For this review, take the finished solid that the model builds, in its own axes (mm). Coordinates: 2 decimals unless noted, no trailing zeros. Loops run counter-clockwise (first coordinate to the right, second up) from the corner with the lowest first, then second, coordinate; pieces in that order, holes last. Notation, with made-up numbers: (-23.75, 26) - (-13.75, 26) arc R16 ccw to (-13.75, 53) - close; hole circle Ø5 at (12, -12). An arc over 180 degrees is marked (long way). One line per item, written item: value. Start each with the question number.
1. Insertion check: pin 1 (4 mm diameter, centred on y = 66.5, z = -1.5, fed in from -X); pin 2 (4 mm diameter, centred on x = -78, z = -1.5, fed in from +Y); pin 3 (1.5 mm diameter, centred on x = -76, z = -1.5, fed in from -Y). Each pin has a flat end and moves straight along its axis. Give the tip position at first contact, or say it passes through.
2. To check wall thickness, follow line 1 (Y direction, x = -69, z = -4); line 2 (Y direction, x = -26, z = -4); line 3 (Z direction, x = 11, y = -23). State the ranges of each line that lie inside material, in increasing order. Write a range as from..to.
3. Take a section at B-B, the plane y = -48.5. State the section outline as (x, z) points.
4. Take a section at C-C, the plane y = 38.5. State the section outline as (x, z) points, and give its area (3 significant figures).
5. Take a section at A-A, the plane x = 58. State the section outline as (y, z) points.
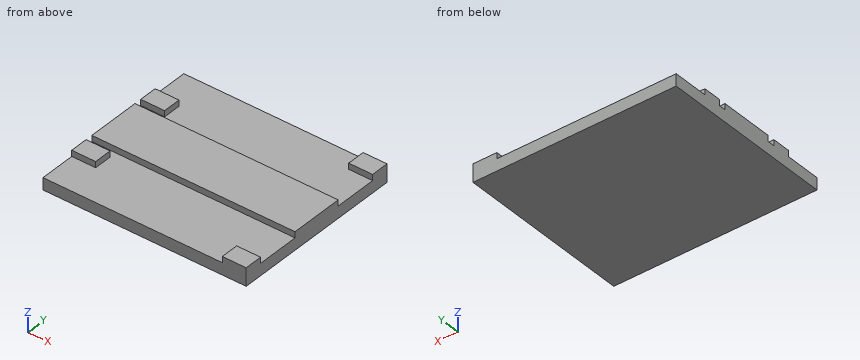
Solid Edge part; units mm, degrees
sketch "Sketch1" plane through (0, 0, 0) normal (0, 0, 1) x (1, 0, 0)
  line L0 (-85, -73.5) -> (85, -73.5)
  line L1 (85, -73.5) -> (85, 73.5)
  line L2 (85, 73.5) -> (-85, 73.5)
  line L3 (-85, 73.5) -> (-85, -73.5)
extrude "Protrusion1" add sketch "Sketch1" against normal blind 15
sketch "Sketch2" plane through (0, 0, 0) normal (0, 0, 1) x (1, 0, 0)
  line L0 (-85, -22.5) -> (85, -22.5)
  line L1 (85, -22.5) -> (85, -28.5)
  line L2 (85, -28.5) -> (-85, -28.5)
  line L3 (-85, -28.5) -> (-85, -22.5)
extrude "ExtrudedCutout_1" cut sketch "Sketch2" against normal blind 5
sketch "Sketch3" plane through (0, 25.5, 0) normal (0, 0, 1) x (1, 0, 0)
  line L0 (-85, -3) -> (85, -3)
  line L1 (85, -3) -> (85, 3)
  line L2 (85, 3) -> (-85, 3)
  line L3 (-85, 3) -> (-85, -3)
extrude "ExtrudedCutout_2" cut sketch "Sketch3" against normal blind 5
sketch "Sketch4" plane through (0, -51, 0) normal (0, 0, 1) x (1, 0, 0)
  line L0 (85, 22.5) -> (-65, 22.5)
  line L1 (-65, 22.5) -> (-65, -22.5)
  line L2 (-65, -22.5) -> (65, -22.5)
  line L3 (65, -22.5) -> (65, -7.5)
  line L4 (65, -7.5) -> (85, -7.5)
  line L5 (85, -7.5) -> (85, 22.5)
extrude "ExtrudedCutout_3" cut sketch "Sketch4" against normal blind 5
sketch "Sketch5" plane through (-75, -51, 0) normal (0, 0, 1) x (1, 0, 0)
  line L0 (-10, 7.5) -> (10, 7.5)
  line L1 (10, 7.5) -> (10, -22.5)
  line L2 (10, -22.5) -> (-10, -22.5)
  line L3 (-10, -22.5) -> (-10, 7.5)
extrude "ExtrudedCutout_4" cut sketch "Sketch5" against normal blind 5
sketch "Sketch6" plane through (0, 51, 0) normal (0, 0, 1) x (1, 0, 0)
  line L0 (-85, 22.5) -> (-85, -7.5)
  line L1 (-85, -7.5) -> (-65, -7.5)
  line L2 (-65, -7.5) -> (-65, -22.5)
  line L3 (-65, -22.5) -> (85, -22.5)
  line L4 (85, -22.5) -> (85, 7.5)
  line L5 (85, 7.5) -> (65, 7.5)
  line L6 (65, 7.5) -> (65, 22.5)
  line L7 (65, 22.5) -> (-85, 22.5)
extrude "ExtrudedCutout_5" cut sketch "Sketch6" against normal blind 5
Solutions:
1. pin 1: x = 65
1. pin 2: y = 43.5
1. pin 3: y = -43.5
2. line 1: -43.5..-28.5, -22.5..22.5, 28.5..43.5
2. line 2: -22.5..22.5
2. line 3: -15..-5
3. outline: (-85, -15) - (85, -15) - (85, -5) - (-85, -5) - close
4. outline: (-85, -15) - (85, -15) - (85, -5) - (-65, -5) - (-65, 0) - (-85, 0) - close
4. area: 1,800 mm2
5. outline: (-73.5, -15) - (73.5, -15) - (73.5, -5) - (22.5, -5) - (22.5, 0) - (-22.5, 0) - (-22.5, -5) - (-73.5, -5) - close
